```python
from build123d import *

# Parameters (mm, degrees)
F1_DEPTH = 2
F0_W     = 71.5
F0_H     = 12.5
F2_DEPTH = 6
F3_DEPTH = 5
F4_DEPTH = 5


with BuildPart() as f1:
    # F0 (on Top) → F1 (new body)
    with BuildSketch(Plane.XY):
        with BuildLine():
            Line((-71, 10.5), (-71, -10.5))
            ThreePointArc((-71, -10.5), (-70.1213203436, -12.6213203436), (-68, -13.5))
            Line((-68, -13.5), (68, -13.5))
            ThreePointArc((68, -13.5), (70.1213203436, -12.6213203436), (71, -10.5))
            Line((71, -10.5), (71, 10.5))
            ThreePointArc((71, 10.5), (70.1213203436, 12.6213203436), (68, 13.5))
            Line((68, 13.5), (-68, 13.5))
            ThreePointArc((-68, 13.5), (-70.1213203436, 12.6213203436), (-71, 10.5))
        make_face()
        with BuildLine():
            Line((58.5, -10.5), (-58.5, -10.5))
            ThreePointArc((-58.5, -10.5), (-65.9246212025, -7.4246212025), (-69, 0))
            ThreePointArc((-69, 0), (-65.9246212025, 7.4246212025), (-58.5, 10.5))
            Line((-58.5, 10.5), (58.5, 10.5))
            ThreePointArc((58.5, 10.5), (65.9246212025, 7.4246212025), (69, 0))
            ThreePointArc((69, 0), (65.9246212025, -7.4246212025), (58.5, -10.5))
        make_face(mode=Mode.SUBTRACT)
    extrude(amount=F1_DEPTH)



with BuildPart() as f2:
    # F0 (on Top) → F2 (new body)
    with BuildSketch(Plane.XY):
        with BuildLine():
            ThreePointArc((-68, 0), (-65.2175144213, -6.7175144213), (-58.5, -9.5))
            Line((-58.5, -9.5), (58.5, -9.5))
            ThreePointArc((58.5, -9.5), (65.2175144213, -6.7175144213), (68, 0))
            ThreePointArc((68, 0), (65.2175144213, 6.7175144213), (58.5, 9.5))
            Line((58.5, 9.5), (-58.5, 9.5))
            ThreePointArc((-58.5, 9.5), (-65.2175144213, 6.7175144213), (-68, 0))
        make_face()
        with BuildLine():
            ThreePointArc((-63.5, 0), (-62.0355339059, 3.5355339059), (-58.5, 5))
            ThreePointArc((-58.5, 5), (-54.9644660941, 3.5355339059), (-53.5, 0))
            ThreePointArc((-53.5, 0), (-54.9644660941, -3.5355339059), (-58.5, -5))
            ThreePointArc((-58.5, -5), (-62.0355339059, -3.5355339059), (-63.5, 0))
        make_face(mode=Mode.SUBTRACT)
        Rectangle(F0_W, F0_H, mode=Mode.SUBTRACT)
        with BuildLine():
            ThreePointArc((53.5, 0), (54.9644660941, 3.5355339059), (58.5, 5))
            ThreePointArc((58.5, 5), (62.0355339059, 3.5355339059), (63.5, 0))
            ThreePointArc((63.5, 0), (62.0355339059, -3.5355339059), (58.5, -5))
            ThreePointArc((58.5, -5), (54.9644660941, -3.5355339059), (53.5, 0))
        make_face(mode=Mode.SUBTRACT)
    extrude(amount=F2_DEPTH)


with BuildPart() as f1_1:
    add(f1.part)

    add(f2.part)  # F3 merges F2
    # F0 (on Top) → F3 (join)
    with BuildSketch(Plane.XY):
        with BuildLine():
            ThreePointArc((-69, 0), (-65.9246212025, -7.4246212025), (-58.5, -10.5))
            Line((-58.5, -10.5), (58.5, -10.5))
            ThreePointArc((58.5, -10.5), (65.9246212025, -7.4246212025), (69, 0))
            ThreePointArc((69, 0), (65.9246212025, 7.4246212025), (58.5, 10.5))
            Line((58.5, 10.5), (-58.5, 10.5))
            ThreePointArc((-58.5, 10.5), (-65.9246212025, 7.4246212025), (-69, 0))
        make_face()
        with BuildLine():
            Line((58.5, -9.5), (-58.5, -9.5))
            ThreePointArc((-58.5, -9.5), (-65.2175144213, -6.7175144213), (-68, 0))
            ThreePointArc((-68, 0), (-65.2175144213, 6.7175144213), (-58.5, 9.5))
            Line((-58.5, 9.5), (58.5, 9.5))
            ThreePointArc((58.5, 9.5), (65.2175144213, 6.7175144213), (68, 0))
            ThreePointArc((68, 0), (65.2175144213, -6.7175144213), (58.5, -9.5))
        make_face(mode=Mode.SUBTRACT)
    extrude(amount=F3_DEPTH)

    # F0 (on Top) → F4 (join)
    with BuildSketch(Plane.XY):
        with BuildLine():
            ThreePointArc((-53.5, 0), (-54.9644660941, 3.5355339059), (-58.5, 5))
            ThreePointArc((-58.5, 5), (-62.0355339059, 3.5355339059), (-63.5, 0))
            ThreePointArc((-63.5, 0), (-62.0355339059, -3.5355339059), (-58.5, -5))
            ThreePointArc((-58.5, -5), (-54.9644660941, -3.5355339059), (-53.5, 0))
        make_face()
        with BuildLine():
            ThreePointArc((63.5, 0), (62.0355339059, 3.5355339059), (58.5, 5))
            ThreePointArc((58.5, 5), (54.9644660941, 3.5355339059), (53.5, 0))
            ThreePointArc((53.5, 0), (54.9644660941, -3.5355339059), (58.5, -5))
            ThreePointArc((58.5, -5), (62.0355339059, -3.5355339059), (63.5, 0))
        make_face()
    extrude(amount=F4_DEPTH)


solid = f1_1.part
```
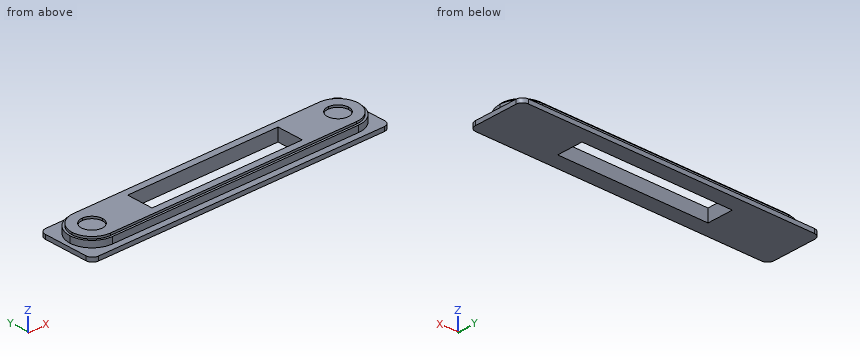
Geometry check sheet. Reference: the model listing, model coordinates, mm. Round coordinates to 2 decimals unless told otherwise and drop trailing zeros. Order: outer loops, then holes, each group sorted by start corner. A loop starts at its lowest first (then second) coordinate and runs counter-clockwise, first axis right, second up. Notation, with made-up numbers: (82.25, 35) - (127.25, 35) arc R18 ccw to (127.25, 68) - close; hole circle Ø8 at (-20.75, -14). An arc over 180 degrees is marked (long way). Use a Markdown table: item, result. Add a question column.
1) Gauge pin test, flat ends, axial feed: P1, Ø1.8, axis at x = 17.5, z = 3.5, coming from the +Y side; P2, Ø3, axis at x = -61, y = 0, coming from the +Z side; P3, Ø1, axis at y = 8, z = 3.5, coming from the -X side; P4, Ø10.5, axis at x = 8.5, y = 0, coming from the +Z side. Record the tip position at first contact, or that the pin passes through.
2) Section check D-D (y = -7.75). Record the cut outline in (x, z).
3) Section check B-B (z = 2.9). Record the cut outline in (x, y).
4) Thickness scan on line 1 along Y through (x, z) = (-4.5, 4); line 2 along X through (y, z) = (-2.25, 0.8); line 3 along Y through (x, z) = (-32.5, 5.75). Record the ranges inside material, lowest first.
5) Section check A-A (x = -8.5). Record the cut outline in (y, z), then the cut area to 3 significant figures.
6) Section check C-C (x = 38). Record the cut outline in (y, z), then the cut area to 3 significant figures.
Established:
| question | item | result |
|---|---|---|
| 1 | P1 | y = 10.5 |
| 1 | P2 | z = 5 |
| 1 | P3 | x = -65.85 |
| 1 | P4 | through |
| 2 | outline | (-71, 0) - (71, 0) - (71, 2) - (65.58, 2) - (65.58, 5) - (63.99, 5) - (63.99, 6) - (-63.99, 6) - (-63.99, 5) - (-65.58, 5) - (-65.58, 2) - (-71, 2) - close |
| 3 | outline | (-58.5, -10.5) - (58.5, -10.5) arc R10.5 ccw to (58.5, 10.5) - (-58.5, 10.5) arc R10.5 ccw to start; hole (-35.75, -6.25) - (35.75, -6.25) - (35.75, 6.25) - (-35.75, 6.25) - close |
| 4 | line 1 | -10.5 to -6.25, 6.25 to 10.5 |
| 4 | line 2 | -71 to -35.75, 35.75 to 71 |
| 4 | line 3 | -9.5 to -6.25, 6.25 to 9.5 |
| 5 | outline | (-13.5, 0) - (-6.25, 0) - (-6.25, 6) - (-9.5, 6) - (-9.5, 5) - (-10.5, 5) - (-10.5, 2) - (-13.5, 2) - close; (6.25, 0) - (13.5, 0) - (13.5, 2) - (10.5, 2) - (10.5, 5) - (9.5, 5) - (9.5, 6) - (6.25, 6) - close |
| 5 | area | 61.0 mm2 |
| 6 | outline | (-13.5, 0) - (13.5, 0) - (13.5, 2) - (10.5, 2) - (10.5, 5) - (9.5, 5) - (9.5, 6) - (-9.5, 6) - (-9.5, 5) - (-10.5, 5) - (-10.5, 2) - (-13.5, 2) - close |
| 6 | area | 136 mm2 |
